Can you work these out from the model? Positions are in its coordinate system, mm. A direction names the side the tool comes from. Give positions to 0.01 mm unless a question says otherwise; leave off trailing zeros. Loops run counter-clockwise (first coordinate to the right, second up) from the corner with the lowest first, then second, coordinate; pieces in that order, holes last. Notation, with made-up numbers: (25, -13) -> (56, -13) arc R20 cw to (56, 22) -> close; hole circle Ø6 at (61, 33.25). An arc over 180 degrees is marked (long way). Return JSON: item names as keys, results as strings. Group by question number.
Q1. I need wall thicknesses on line 1 along X through (y, z) = (-1.75, -33.5); line 2 along Z through (x, y) = (-3.75, 3.25); line 3 along X through (y, z) = (1.5, -29). Which ranges of each line are inside material? Lowest first, please. Write a range as [from, to].
Q2. Suppose I cut it at D-D, the plane z = 0. Please give me the cut outline in (x, y).
Q3. Will this pin go through, and if not, where does the flat tip stop? pin 1 (5.5 mm diameter, centred on x = -0.5, z = -17, fed in from -Y).
Q4. Which directions (+Z, -Z, +X, -X, +Y, -Y) give clear straight access to the entire face, cutting with the end or side of a thin tool? Please do faces 5 (the flat face through (6.2, 4, -30)), 6 (the cylindrical face through (7, 0, -28)), 7 (the flat face through (12, 1, -25)), 8 (the flat face through (0, 3, -42)).
Q5. Thinking about a two-plate mould opening in Z: for faces 1 (the cylindrical face through (9.594, 0.563, 9.719)), 2 (the cylindrical face through (-10.073, 0.481, -32.528)), 3 (the flat face through (0, 0, -55)), 4 (the flat face through (0, -2, -14)), which applies, pulls with the +Z half, pulls with the -Z half, needs draft (parallel to the pull), parting line crosses it, or undercut?
Q6. Suppose I cut it at C-C, the plane y = 4. Please give me the cut outline in (x, z), and give its area (3 significant figures).
Q7. Suppose I cut it at A-A, the plane y = 0. Count the separate pieces of the cut face and the enclosed holes in it, and give its area (3 significant figures).
```python
from build123d import *

# Parameters (mm, degrees)
SKETCH_1_W          = 67
SKETCH_1_H          = 9
EXTRUDE_1_DEPTH     = 12
SKETCH_2_R          = 6.7
CUT_EXTRUDE_1_DEPTH = 5
SKETCH_4_R          = 3.2
CUT_EXTRUDE_3_DEPTH = 57.515484604
SKETCH_3_W          = 12.4
SKETCH_3_H          = 23.085257288
CUT_EXTRUDE_2_DEPTH = 58.008771255
SKETCH_5_W          = 12.4
SKETCH_5_H          = 32.914742712
CUT_EXTRUDE_4_DEPTH = 5
SKETCH_6_R          = 0.855484329
CUT_EXTRUDE_5_DEPTH = 57.515484604
FILLET_1_R          = 8
SKETCH_7_R          = 1.6
CUT_EXTRUDE_6_DEPTH = 61.216276869
SKETCH_8_R          = 3
CUT_EXTRUDE_7_DEPTH = 2


with BuildPart() as part:
    # 草图1 → 凸台-拉伸1 (new, symmetric)
    with BuildSketch(Plane(origin=(0, 0, 0), x_dir=(0, 0, -1), z_dir=(1, 0, 0))):
        with Locations((21.5, 0.5)):
            Rectangle(SKETCH_1_W, SKETCH_1_H)
    extrude(amount=EXTRUDE_1_DEPTH, both=True)

    # 草图2 → 切除-拉伸1 (cut)
    with BuildSketch(Plane(origin=(0, -4, 0), x_dir=(1, 0, 0), z_dir=(0, 1, 0))):
        with Locations(Location((0, 0, 0), (0, 0, 270))):
            Circle(SKETCH_2_R)
    extrude(amount=CUT_EXTRUDE_1_DEPTH, mode=Mode.SUBTRACT)

    # 草图4 → 切除-拉伸3 (cut, through all)
    with BuildSketch(Plane.XZ.offset(-1)):
        with Locations(Location((0, 0, 0), (0, 0, 270))):
            Circle(SKETCH_4_R)
    extrude(amount=-CUT_EXTRUDE_3_DEPTH, mode=Mode.SUBTRACT)

    # 草图3 → 切除-拉伸2 (cut, through all)
    with BuildSketch(Plane(origin=(0, 5, 0), x_dir=(1, 0, 0), z_dir=(0, 1, 0))):
        with Locations((0, 30.457371356)):
            Rectangle(SKETCH_3_W, SKETCH_3_H)
    extrude(amount=-CUT_EXTRUDE_2_DEPTH, mode=Mode.SUBTRACT)

    # 草图5 → 切除-拉伸4 (cut)
    with BuildSketch(Plane.XZ.offset(4)):
        with Locations((0, -30.457371356)):
            Rectangle(SKETCH_5_W, SKETCH_5_H)
    extrude(amount=-CUT_EXTRUDE_4_DEPTH, mode=Mode.SUBTRACT)

    # 草图6 → 切除-拉伸5 (cut, through all)
    with BuildSketch(Plane.XZ.offset(-1)):
        with Locations(Location((0, -15.957371356, 0), (0, 0, 270))):
            Circle(SKETCH_6_R)
        with Locations(Location((0, -44.957371356, 0), (0, 0, 90))):
            Circle(SKETCH_6_R)
    extrude(amount=-CUT_EXTRUDE_5_DEPTH, mode=Mode.SUBTRACT)

    # 圆角1
    fillet_1_edges = [part.edges().sort_by_distance(p)[0] for p in [
        (12, 0.5, 12),
        (-12, 0.5, 12),
    ]]
    fillet(fillet_1_edges, radius=FILLET_1_R)

    # 草图7 → 切除-拉伸6 (cut, through all)
    with BuildSketch(Plane(origin=(12, 0, 0), x_dir=(0, 0, -1), z_dir=(1, 0, 0))):
        with Locations((51.001572261, 0)):
            Circle(SKETCH_7_R)
        with Locations((31.001572261, 0)):
            Circle(SKETCH_7_R)
    extrude(amount=-CUT_EXTRUDE_6_DEPTH, mode=Mode.SUBTRACT)

    # 草图8 → 切除-拉伸7 (cut)
    with BuildSketch(Plane(origin=(-6.2, 0, 0), x_dir=(0, 0, -1), z_dir=(1, 0, 0))):
        with Locations((31.001572261, 0)):
            Circle(SKETCH_8_R)
    cut_extrude_7 = extrude(amount=-CUT_EXTRUDE_7_DEPTH, mode=Mode.SUBTRACT)

    # 镜向1: 切除-拉伸7 across plane
    add(cut_extrude_7.mirror(Plane(origin=(0, 0, 0), x_dir=(0, 0, 1), z_dir=(1, 0, 0))), mode=Mode.SUBTRACT)


solid = part.part
```
Ans:
{
 "1": {"line 1": "x = [-12, -6.2], [6.2, 12]", "line 2": "z = [-55, -42], [-18.91, 12]", "line 3": "x = [-12, -8.2], [8.2, 12]"},
 "2": {"outline": "(-12, -4) -> (-6.7, -4) -> (-6.7, 1) -> (-3.2, 1) -> (-3.2, 5) -> (-12, 5) -> close; (3.2, 1) -> (6.7, 1) -> (6.7, -4) -> (12, -4) -> (12, 5) -> (3.2, 5) -> close"},
 "3": {"pin 1": "stops at y = 1"},
 "4": {"face 5": "-Y", "face 6": "none", "face 7": "+Z, -Z, +X, +Y, -Y", "face 8": "+Y, -Y"},
 "5": {"face 1": "pulls with the +Z half", "face 2": "undercut", "face 3": "pulls with the -Z half", "face 4": "undercut"},
 "6": {"outline": "(-12, -55) -> (12, -55) -> (12, 4) arc R8 ccw to (4, 12) -> (-4, 12) arc R8 ccw to (-12, 4) -> close; hole (-6.2, -42) -> (6.2, -42) -> (6.2, -18.91) -> (-6.2, -18.91) -> close; hole circle Ø6.4 at (0, 0); hole circle Ø1.71 at (0, -44.96); hole circle Ø1.71 at (0, -15.96)", "area": "1,260 mm^2"},
 "7": {"separate pieces": "3", "enclosed holes": "1", "area": "906 mm^2"}
}
